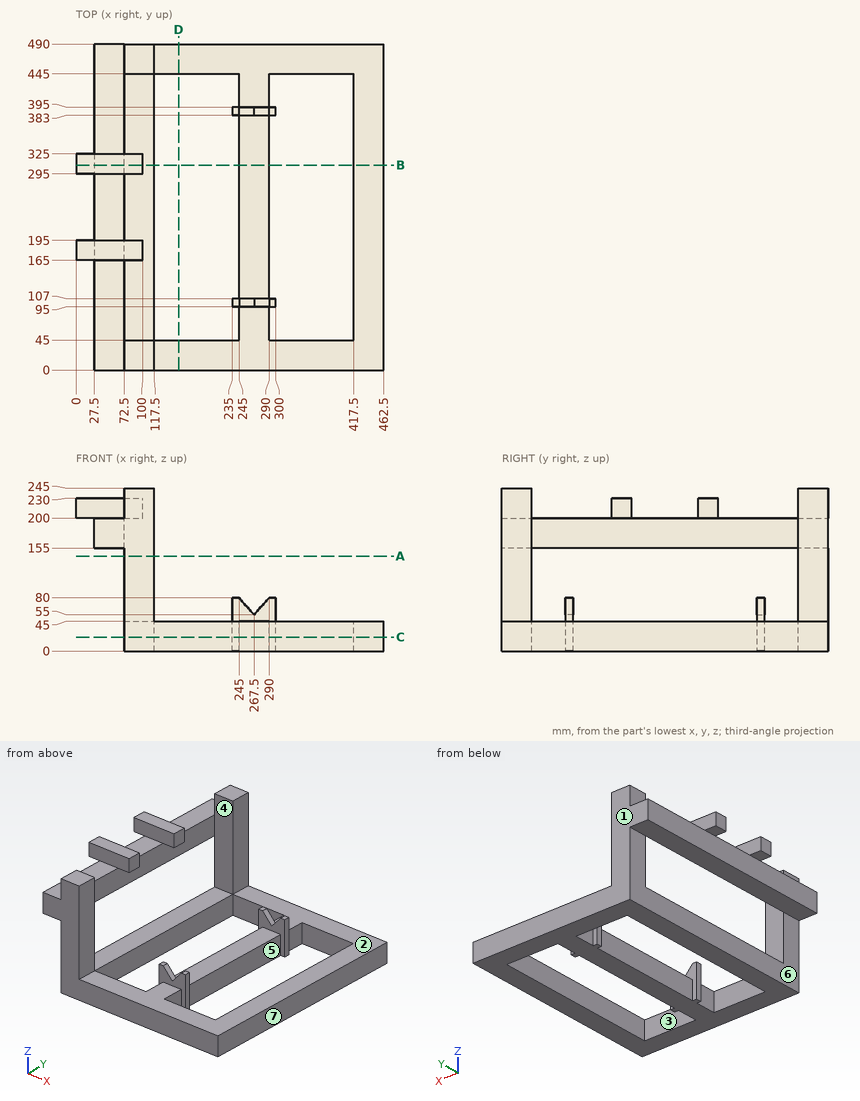
Verification items for this drawing (mm, ordinates from the low corner). A direction names the side the tool comes from. Coordinates: 2 decimals unless noted, no trailing zeros. Write each loop counter-clockwise with the first axis right and the second up, starting at its lowest first coordinate (ties: lowest second). Pieces come first, ordered by that corner, then holes. Notation, with made-up numbers: M 26.25,61 L 37.25,61 A20 cw 37.25,91 Z; hole C -30,6.25 d6. An arc over 180 degrees is marked long. Answer as a JSON object with one key per item and string values.
1. Scan lines: L1, parallel to X at y = 108, z = 10; L2, parallel to Y at x = 180.5, z = 18; L3, parallel to Z at x = 233, y = 32. Record each from-to range of solid material in increasing order.
Answers below:
{"L1": "x = 72.5 to 117.5, 245 to 290, 417.5 to 462.5", "L2": "y = 0 to 45, 445 to 490", "L3": "z = 0 to 45"}
2. Section check C-C, the plane z = 21. Enter the section's corners in (x, y).
Answers below:
{"outline": "M 72.5,0 L 462.5,0 L 462.5,490 L 72.5,490 Z; hole M 117.5,45 L 245,45 L 245,95 L 235,95 L 235,107 L 245,107 L 245,383 L 235,383 L 235,395 L 245,395 L 245,445 L 117.5,445 Z; hole M 290,45 L 417.5,45 L 417.5,445 L 290,445 L 290,395 L 300,395 L 300,383 L 290,383 L 290,107 L 300,107 L 300,95 L 290,95 Z"}
3. Tool access check on the marked faces 4, 5, 6 and 7. Record the directions out of +Z, -Z, +X, -X, +Y, -Y that give a thin tool (end or side, any length) a straight path to the whole face; none if there is none.
Answers below:
{"face 4": "+Z, +X", "face 5": "+Z, -Z", "face 6": "-Z, -X, +Y, -Y", "face 7": "+Z, -Z, +X, +Y, -Y"}
4. Section check B-B, the plane y = 308. Enter the section's corners in (x, z).
Answers below:
{"outline": "M 0,200 L 27.5,200 L 27.5,155 L 72.5,155 L 72.5,200 L 100,200 L 100,230 L 0,230 Z; M 72.5,0 L 117.5,0 L 117.5,45 L 72.5,45 Z; M 245,0 L 290,0 L 290,45 L 245,45 Z; M 417.5,0 L 462.5,0 L 462.5,45 L 417.5,45 Z"}
5. Go/stop test with flat-tipped pins: pin 1 Ø8 at (x, y) = (297, 99.5) entering from +Z; pin 2 Ø4 at (y, z) = (107, 80.5) entering from +X; pin 3 Ø13.5 at (x, y) = (45.5, 58) entering from +Z. Record where each tip stops, or that it passes through.
Answers below:
{"pin 1": "stops at z = 80", "pin 2": "stops at x = 300", "pin 3": "stops at z = 200"}
6. Section check A-A, the plane z = 143. Enter the section's corners in (x, y), plus the area to 3 significant figures.
Answers below:
{"outline": "M 72.5,0 L 117.5,0 L 117.5,45 L 72.5,45 Z; M 72.5,445 L 117.5,445 L 117.5,490 L 72.5,490 Z", "area": "4,050 mm²"}
7. Draft check along Y on the marked faces 1, 2 and 3. Enter one of: released by +Y, released by -Y, zero draft, split by the parting line, or undercut.
Answers below:
{"face 1": "released by +Y", "face 2": "zero draft", "face 3": "undercut"}
8. Section check D-D, the plane x = 154. Enter the section's corners in (y, z), plus the area to 3 significant figures.
Answers below:
{"outline": "M 0,0 L 45,0 L 45,45 L 0,45 Z; M 445,0 L 490,0 L 490,45 L 445,45 Z", "area": "4,050 mm²"}
